Can you work these out from the model? Positions are in its coordinate system, mm. A direction names the side the tool comes from. Coordinates: 2 decimals unless noted, no trailing zeros. Order: outer loops, then holes, each group sorted by start corner. A loop starts at its lowest first (then second) coordinate and runs counter-clockwise, first axis right, second up.
Autodesk Inventor part; units mm, degrees
ref_plane "YZ Plane" through (0, 0, 0) normal (1, 0, 0) x (0, 1, 0)
ref_plane "XZ Plane" through (0, 0, 0) normal (0, 1, 0) x (-1, 0, 0)
ref_plane "XY Plane" through (0, 0, 0) normal (0, 0, 1) x (1, 0, 0)
sketch "スケッチ1" plane through (0, 0, 0) normal (1, 0, 0) x (0, 1, 0)
  line L0 (0, 0) -> (1.25, 0)
  line L1 (1.25, 0) -> (1.25, -5)
  line L2 (1.25, -5) -> (0, -5)
  line L3 (0, -5) -> (0, 0)
  line L4 (0, -5) -> (2.25, -5)
  line L5 (2.25, -5) -> (2.25, -7.5)
  line L6 (2.25, -7.5) -> (0, -7.5)
  line L7 (0, -7.5) -> (0, -5)
  line L8 (2.25, -7.3) -> (2.05, -7.5)
  line L9 (1.25, -0.12) -> (1.13, 0)
  point P0 (2.25, -6.25)
  dimension "d0" = 45
  dimension "d1" = 2.25
  dimension "d2" = 2.5
  dimension "d3" = 5
  dimension "d7" = 1.25
  dimension "d10" = 45
  dimension "d11" = 0.2
  dimension "d12" = 0.12
revolve "回転1" add sketch "スケッチ1" angle 360 about axis through (0, 0, -5) along (0, 0, 1) contours L0 L9 L1 L2 L3 | L2 L4 L5 L8 L6 L7
thread "ねじ2"
properties part number "M2-5_5mm" material "ステンレス鋼"
1. On a 3-axis mill with a long thin cutter (end or side, diameter ignored), from which of +Z, -Z, +X, -X, +Y, -Y can I reach the whole of each face in a straight line? I mean faces 1 (the flat face through (1, 1, -5)), 2 (the flat face through (0, 0, -7.5)). Say none if no direction works.
Completed:
face 1: +Z
face 2: -Z, +X, -X, +Y, -Y
2. Imagine slicing it at D-D on z = -6.75. Please give me the cut outline in (x, y).
Completed:
outline: circle Ø4.5 at (0, 0)
3. Please list where these lines run through material, in increasing order: probe 1 along Z at (x, y) = (-1.9, 0.2); probe 2 along Y at (x, z) = (0.9, -4); probe 3 along X at (y, z) = (2, -6.5).
Completed:
probe 1: z = -7.5 to -5
probe 2: y = -0.87 to 0.87
probe 3: x = -1.03 to 1.03
4. Imagine slicing it at A-A on y = 0. Please give me the cut outline in (x, z).
Completed:
outline: (-2.25, -7.3) - (-2.05, -7.5) - (2.05, -7.5) - (2.25, -7.3) - (2.25, -5) - (1.25, -5) - (1.25, -0.12) - (1.13, 0) - (-1.13, 0) - (-1.25, -0.12) - (-1.25, -5) - (-2.25, -5) - close
5. I'm going to push flat-ended pins straight in: pin 1 (2 mm diameter, centred on y = 1, z = -2, fed in from +X); pin 2 (1 mm diameter, centred on x = -1, z = -2.5, fed in from -Y). Where does each tip first touch, or does it pass through?
Completed:
pin 1: stops at x = 1.25
pin 2: stops at y = -1.15
6. Imagine slicing it at C-C on z = -3.5. Please give me the cut outline in (x, y), then the cut area to 3 significant figures.
Completed:
outline: circle Ø2.5 at (0, 0)
area: 4.91 mm2
